Input: part model. Units: mm. Frame: model coordinates. Face numbers are marked on the shaded views. A direction names the side the tool comes from. Give positions to 0.01 mm unless a question says otherwise; leave off trailing zeros. Order: outer loops, then holes, each group sorted by start corner. A loop starts at its lowest first (then second) coordinate and runs counter-clockwise, first axis right, second up. Notation, with made-up numbers: (-22, 42) - (9, 42) arc R33 cw to (9, 73) - close; hole circle Ø1 at (0, 68). An arc over 180 degrees is marked (long way). Answer in a Markdown table with one row per item. Add a question column.
1. Contact query for flat-ended pins moving along their axis: pin 1 (1.5 mm diameter, centred on x = 13.5, y = 1, fed in from +Z); pin 2 (6 mm diameter, centred on x = -19, z = 3.5, fed in from -Y); pin 3 (1.5 mm diameter, centred on y = 3.5, z = 0.5, fed in from +X). Output: stop coordinate, or through.
2. Section query C-C on x = -1.5. Return loops of the section in (y, z) (3 decimals).
3. Section query A-A on z = 5. Return loops of the section in (x, y) (3 decimals), and give its area (3 significant figures).
4. Ray query, line 1 (X direction, y = 4.5, z = 11.5) (3 decimals); line 2 (Z direction, x = 17.5, y = 0.25) (3 decimals); line 3 (X direction, y = -0.25, z = -0.5). Return the intervals inside material, ascending. Write a range as [from, to].
5. Access query for the marked faces 5 and 6. Directions: +Z, -Z, +X, -X, +Y, -Y. A direction counts if a zero-diameter tool reaches every point of the face in a straight line with its end or side. Return the directions, or none.
6. Section query D-D on z = 0.5. Return loops of the section in (x, y).
7. Mould query, pull axis X, two halves, no side actions, for the marked faces 1, 2, 3 and 4. Classes: released by +X, released by -X, zero draft, split by the parting line, or undercut.
8. Section query B-B on y = 4. Return loops of the section in (x, z) (3 decimals), and give its area (3 significant figures).
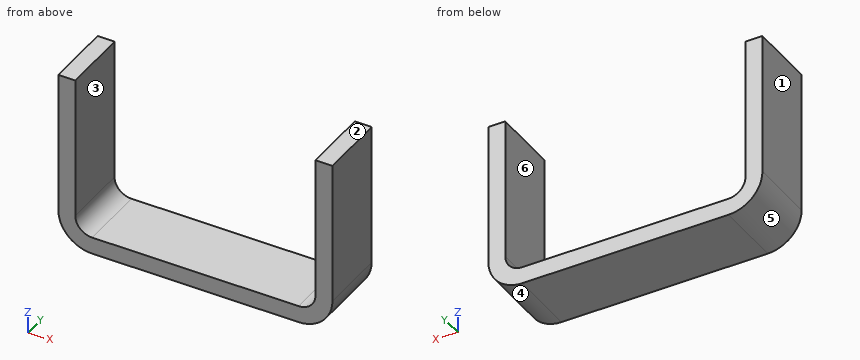
```python
from build123d import *

# Parameters (mm, degrees)
F1_DEPTH = 6.35
F2_R     = 3.175
F3_R     = 6.35


with BuildPart() as f1:
    # F0 (on Front) → F1 (new body, symmetric)
    with BuildSketch(Plane.XZ):
        Polygon((22.5, 0), (0, 0), (-22.5, 0), (-22.5, 30), (-25.675, 30), (-25.675, -3.175), (0, -3.175), (25.675, -3.175), (25.675, 30), (22.5, 30), align=None)
    extrude(amount=F1_DEPTH, both=True)

    # F2
    f2_edges = [f1.edges().sort_by_distance(p)[0] for p in [
        (22.5, 0, 0),
        (-22.5, 0, 0),
    ]]
    fillet(f2_edges, radius=F2_R)

    # F3
    f3_edges = [f1.edges().sort_by_distance(p)[0] for p in [
        (-25.675, 0, -3.175),
        (25.675, 0, -3.175),
    ]]
    fillet(f3_edges, radius=F3_R)


solid = f1.part
```
Answer:
| question | item | result |
|---|---|---|
| 1 | pin 1 | stops at z = 0 |
| 1 | pin 2 | passes through |
| 1 | pin 3 | stops at x = 25.38 |
| 2 | outline | (-6.35, -3.175) - (6.35, -3.175) - (6.35, 0) - (-6.35, 0) - close |
| 3 | outline | (-25.675, -6.35) - (-22.5, -6.35) - (-22.5, 6.35) - (-25.675, 6.35) - close; (22.5, -6.35) - (25.675, -6.35) - (25.675, 6.35) - (22.5, 6.35) - close |
| 3 | area | 80.6 mm² |
| 4 | line 1 | x = [-25.675, -22.5], [22.5, 25.675] |
| 4 | line 2 | z = [-3.175, 0] |
| 4 | line 3 | x = [-24.5, 24.5] |
| 5 | face 5 | -Z, -X, +Y, -Y |
| 5 | face 6 | +Z, +Y, -Y |
| 6 | outline | (-25.08, -6.35) - (-21.04, -6.35) - (-21.04, 6.35) - (-25.08, 6.35) - close; (21.04, -6.35) - (25.08, -6.35) - (25.08, 6.35) - (21.04, 6.35) - close |
| 7 | face 1 | released by -X |
| 7 | face 2 | zero draft |
| 7 | face 3 | undercut |
| 7 | face 4 | released by +X |
| 8 | outline | (-25.675, 3.175) arc R6.35 ccw to (-19.325, -3.175) - (19.325, -3.175) arc R6.35 ccw to (25.675, 3.175) - (25.675, 30) - (22.5, 30) - (22.5, 3.175) arc R3.175 cw to (19.325, 0) - (-19.325, 0) arc R3.175 cw to (-22.5, 3.175) - (-22.5, 30) - (-25.675, 30) - close |
| 8 | area | 341 mm² |
